Model file for the job. Use its own axes, mm. A direction names the side the tool comes from. Coordinates: 2 decimals unless noted, no trailing zeros. Loops run counter-clockwise (first coordinate to the right, second up) from the corner with the lowest first, then second, coordinate; pieces in that order, holes last. Notation, with made-up numbers: (-4.75, -16) - (10.25, -16) arc R36 ccw to (10.25, 22) - close; hole circle Ø4 at (-20.5, 56.5). An arc over 180 degrees is marked (long way). Write each question's results on one line, items separated by ' | '. Start each with the question number.
```python
from build123d import *

# Parameters (mm, degrees)
SKETCH1_W           = 146
SKETCH1_H           = 105
BOSS_EXTRUDE1_DEPTH = 3
SKETCH2_W           = 3
SKETCH2_H           = 20
CUT_EXTRUDE1_DEPTH  = 10
SKETCH3_R           = 1.7
SKETCH3_W           = 60.4
SKETCH3_H           = 42.72
CUT_EXTRUDE2_DEPTH  = 3
SKETCH5_W           = 3
SKETCH5_H           = 30.32
CUT_EXTRUDE4_DEPTH  = 90.968049884
SKETCH6_R           = 1.6
CUT_EXTRUDE5_DEPTH  = 10


with BuildPart() as part:
    # Sketch1 → Boss-Extrude1 (new body)
    with BuildSketch(Plane(origin=(0, 0, 0), x_dir=(1, 0, 0), z_dir=(0, 1, 0))):
        Rectangle(SKETCH1_W, SKETCH1_H)
    extrude(amount=BOSS_EXTRUDE1_DEPTH)

    # Sketch2 → Cut-Extrude1 (cut)
    with BuildSketch(Plane(origin=(0, 3, 0), x_dir=(1, 0, 0), z_dir=(0, 1, 0))):
        with Locations((-71.5, 16.47)):
            Rectangle(SKETCH2_W, SKETCH2_H)
        with Locations((71.5, 16.47)):
            Rectangle(SKETCH2_W, SKETCH2_H)
        with Locations((-71.5, -29.4)):
            Rectangle(SKETCH2_W, SKETCH2_H)
        with Locations((71.5, -29.4)):
            Rectangle(SKETCH2_W, SKETCH2_H)
    extrude(amount=-CUT_EXTRUDE1_DEPTH, mode=Mode.SUBTRACT)

    # Sketch3 → Cut-Extrude2 (cut)
    with BuildSketch(Plane(origin=(0, 0, 0), x_dir=(-1, 0, 0), z_dir=(0, -1, 0))):
        with Locations(Location((-34, 29.3, 0), (0, 0, 90))):
            Circle(SKETCH3_R)
        with Locations(Location((-34, -7.02, 0), (0, 0, 90))):
            Circle(SKETCH3_R)
        with Locations(Location((34, 29.3, 0), (0, 0, 90))):
            Circle(SKETCH3_R)
        with Locations(Location((34, -7.02, 0), (0, 0, 90))):
            Circle(SKETCH3_R)
        with Locations((0, 11.14)):
            Rectangle(SKETCH3_W, SKETCH3_H)
    extrude(amount=-CUT_EXTRUDE2_DEPTH, mode=Mode.SUBTRACT)

    # Sketch5 → Cut-Extrude4 (cut, through all)
    with BuildSketch(Plane(origin=(0, 0, 0), x_dir=(-1, 0, 0), z_dir=(0, -1, 0))):
        with Locations((31.7, 11.14)):
            Rectangle(SKETCH5_W, SKETCH5_H)
        with Locations((-31.7, 11.14)):
            Rectangle(SKETCH5_W, SKETCH5_H)
    extrude(amount=-CUT_EXTRUDE4_DEPTH, mode=Mode.SUBTRACT)

    # Sketch6 → Cut-Extrude5 (cut)
    with BuildSketch(Plane.XZ):
        with Locations(Location((-66, 2.92, 0), (0, 0, 270))):
            Circle(SKETCH6_R)
        with Locations(Location((66, 2.92, 0), (0, 0, 270))):
            Circle(SKETCH6_R)
    extrude(amount=-CUT_EXTRUDE5_DEPTH, mode=Mode.SUBTRACT)


solid = part.part
```
Q1. Which spindle directions (+Z, -Z, +X, -X, +Y, -Y) get a long thin tool onto all of the face, cutting with end or side? Do faces 1 (the flat face through (73, 1, -39)), 2 (the flat face through (30.2, 1, 7)), 3 (the flat face through (-70, 2, 30)), 4 (the flat face through (70, 2, 30)), 5 (the flat face through (-73, 1, 7)). Say none if no direction does.
Q2. Drill centre lines: L1, parallel to X at y = 1, z = 3; L2, parallel to X at y = 1.25, z = -29.3; L3, parallel to Z at x = 66, y = 0.9. Where is each one in solid material? Low to high. Write a range as from..to.
Q3. Pin check, flat tip, straight feed: pin 1 (2.5 mm diameter, centred on x = -66, z = 2.92, fed in from +Y). Stop position of the tip, or through.
Q4. Cut at B-B (x = 66). List the corners of the cut face in (y, z).
Q5. Cut at D-D (y = 2.35). State how many separate pieces and enclosed holes the cut face has, and give its area (3 significant figures).
Q6. Cut at A-A (z = -19.5). List the corners of the cut face in (x, y), and give its area (3 significant figures).
Q7. Cut at C-C (z = 7.02). List the corners of the cut face in (x, y), and give its area (3 significant figures).
Q8. Mould opens along Z. For faces 6 (the flat face through (-1, 1, -52.5)), 7 (the flat face through (73, 1, 7)), 8 (the cylindrical face through (-35.66, 1.48, 7.39)) say: +Z half, -Z half, draft (parallel to the pull), parting line (faces both ways), or undercut.
Check result:
1) face 1: +Z, -Z, +X, +Y, -Y | face 2: +Y, -Y | face 3: -X, +Y, -Y | face 4: +X, +Y, -Y | face 5: +Z, -Z, -X, +Y, -Y
2) L1: -73..-67.6, -64.4..-33.2, 33.2..64.4, 67.6..73 | L2: -73..-35.7, -32.3..-30.2, 30.2..32.3, 35.7..73 | L3: -52.5..1.32, 4.52..52.5
3) pin 1: through
4) outline: (0, -52.5) - (3, -52.5) - (3, 1.32) - (0, 1.32) - close; (0, 4.52) - (3, 4.52) - (3, 52.5) - (0, 52.5) - close
5) separate pieces: 1 | enclosed holes: 7 | area: 12,300 mm²
6) outline: (-70, 0) - (-33.2, 0) - (-33.2, 3) - (-70, 3) - close; (33.2, 0) - (70, 0) - (70, 3) - (33.2, 3) - close | area: 221 mm²
7) outline: (-73, 0) - (-35.7, 0) - (-35.7, 3) - (-73, 3) - close; (-32.3, 0) - (-30.2, 0) - (-30.2, 3) - (-32.3, 3) - close; (30.2, 0) - (32.3, 0) - (32.3, 3) - (30.2, 3) - close; (35.7, 0) - (73, 0) - (73, 3) - (35.7, 3) - close | area: 236 mm²
8) face 6: -Z half | face 7: draft | face 8: undercut
